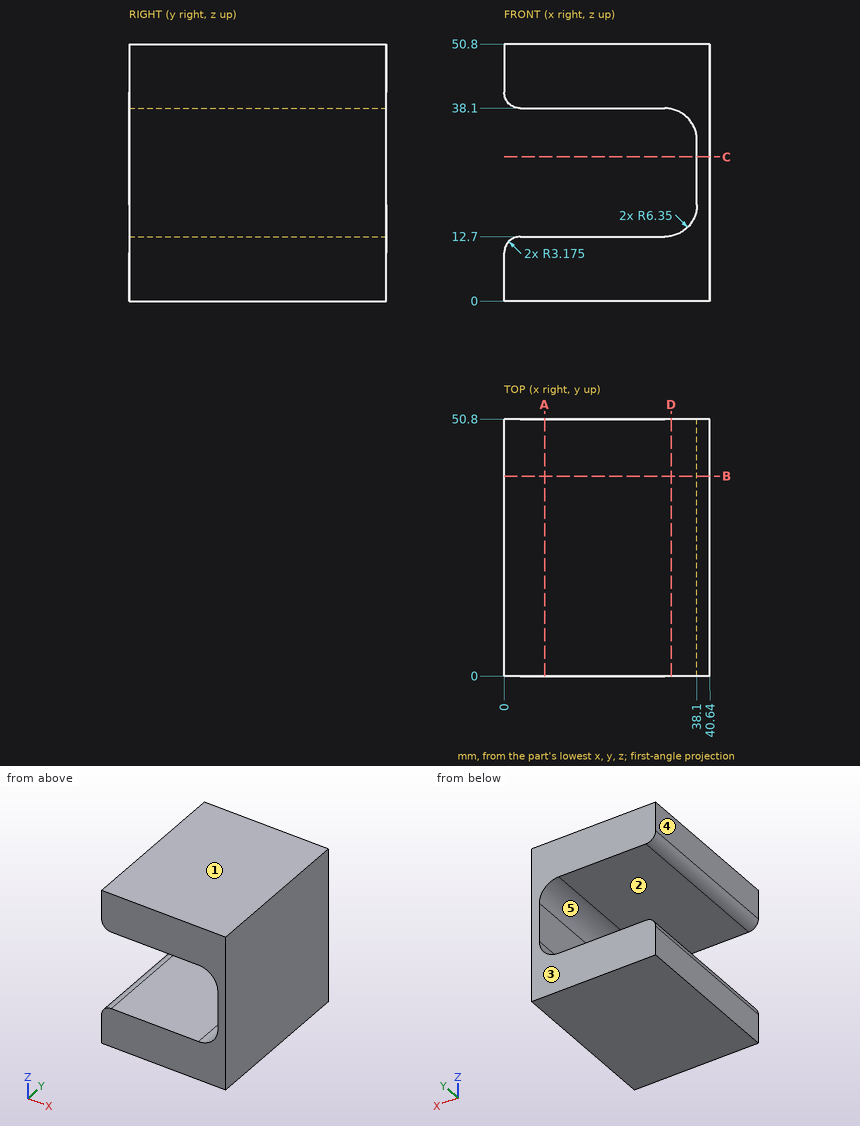
For this review, use the dimensioned drawing (mm, ordinates from the lowest corner) and the shaded views. A direction names the side the tool comes from. Give positions to 0.01 mm unless a question says otherwise; leave off trailing zeros. Order: outer loops, then holes, each group sorted by start corner. A loop starts at its lowest first (then second) coordinate and runs counter-clockwise, first axis right, second up.
1. Tool access review of the marked faces 4 and 5: name each direction out of +Z, -Z, +X, -X, +Y, -Y from which nothing blocks a thin tool from reaching the whole face with its end or side.
Solution:
face 4: +Z, -Z, -X, +Y, -Y
face 5: -X, +Y, -Y
2. Add section B-B, the plane y = 39.5. State the section outline as (x, z) points (3 decimals).
Solution:
outline: (0, 0) - (40.64, 0) - (40.64, 50.8) - (0, 50.8) - (0, 41.275) arc R3.175 ccw to (3.175, 38.1) - (31.75, 38.1) arc R6.35 cw to (38.1, 31.75) - (38.1, 19.05) arc R6.35 cw to (31.75, 12.7) - (3.175, 12.7) arc R3.175 ccw to (0, 9.525) - close
3. Add section A-A, the plane x = 8. State the section outline as (y, z) points, then the cut area to 3 significant figures.
Solution:
outline: (0, 0) - (50.8, 0) - (50.8, 12.7) - (0, 12.7) - close; (0, 38.1) - (50.8, 38.1) - (50.8, 50.8) - (0, 50.8) - close
area: 1,290 mm2
4. Mouldability with a two-part tool opening along Z and no side actions: class the marked faces 1, 2 and 3 as +Z half, -Z half, draft (parallel to the pull), parting line (faces both ways), or undercut.
Solution:
face 1: +Z half
face 2: undercut
face 3: draft
5. To check wall thickness, follow L1, parallel to Z at x = 24.5, y = 5; L2, parallel to X at y = 33.5, z = 31.5; L3, parallel to Z at x = 37, y = 15. State the ranges of each line that lie inside material, in increasing order.
Solution:
L1: z = 0 to 12.7, 38.1 to 50.8
L2: x = 38.1 to 40.64
L3: z = 0 to 15.48, 35.32 to 50.8
6. Add section C-C, the plane z = 28.5. State the section outline as (x, y) points.
Solution:
outline: (38.1, 0) - (40.64, 0) - (40.64, 50.8) - (38.1, 50.8) - close
7. For pin 1 Ø10 at (y, z) = (16, 32.5) entering from -X; pin 2 Ø6.5 at (y, z) = (29.5, 25) entering from -X, all flat-tipped, find the tip position at first contact; note any pin that passes through.
Solution:
pin 1: stops at x = 34.44
pin 2: stops at x = 38.1
8. Add section D-D, the plane x = 33. State the section outline as (y, z) points, then the cut area to 3 significant figures.
Solution:
outline: (0, 0) - (50.8, 0) - (50.8, 12.82) - (0, 12.82) - close; (0, 37.98) - (50.8, 37.98) - (50.8, 50.8) - (0, 50.8) - close
area: 1,300 mm2
